from build123d import *

# Parameters (mm, degrees)
SKETCH_1_W          = 31.8
SKETCH_1_H          = 7.8
EXTRUDE_1_DEPTH     = 3.2
SKETCH_2_R          = 2.4
EXTRUDE_2_DEPTH     = 1.7
SKETCH_3_R          = 2.5
CUT_EXTRUDE_1_DEPTH = 1.8


with BuildPart() as part:
    # Эскиз1 → Бобышка-Вытянуть1 (new body)
    with BuildSketch(Plane(origin=(0, 0, 0), x_dir=(1, 0, 0), z_dir=(0, 1, 0))):
        Rectangle(SKETCH_1_W, SKETCH_1_H)
    extrude(amount=EXTRUDE_1_DEPTH)

    # Эскиз2 → Бобышка-Вытянуть2 (add)
    with BuildSketch(Plane(origin=(0, 3.2, 0), x_dir=(1, 0, 0), z_dir=(0, 1, 0))):
        with Locations(Location((-12, 0, 0), (0, 0, 270))):
            Circle(SKETCH_2_R)
        with Locations(Location((-4.126, 0, 0), (0, 0, 270))):
            Circle(SKETCH_2_R)
        with Locations(Location((3.748, 0, 0), (0, 0, 270))):
            Circle(SKETCH_2_R)
        with Locations(Location((11.622, 0, 0), (0, 0, 270))):
            Circle(SKETCH_2_R)
    extrude(amount=EXTRUDE_2_DEPTH)

    # Эскиз3 → Вырез-Вытянуть1 (cut)
    with BuildSketch(Plane.XZ):
        with Locations(Location((-12, 0, 0), (0, 0, 270))):
            Circle(SKETCH_3_R)
        with Locations(Location((-4.126, 0, 0), (0, 0, 270))):
            Circle(SKETCH_3_R)
        with Locations(Location((3.748, 0, 0), (0, 0, 270))):
            Circle(SKETCH_3_R)
        with Locations(Location((11.622, 0, 0), (0, 0, 270))):
            Circle(SKETCH_3_R)
    extrude(amount=-CUT_EXTRUDE_1_DEPTH, mode=Mode.SUBTRACT)


solid = part.part
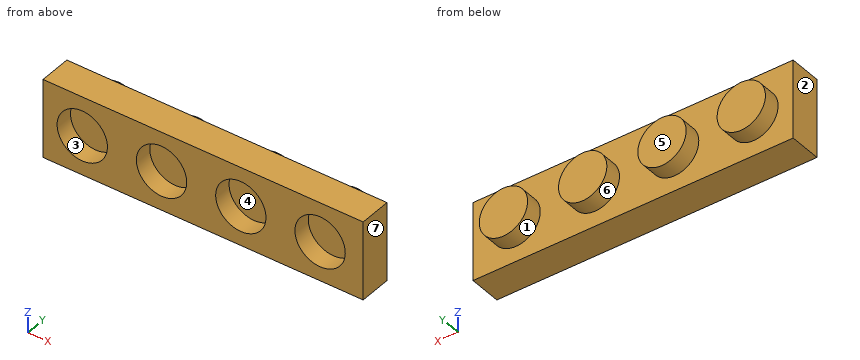
Source: CAD feature listing. Evaluate the final solid. Frame: model axes, mm. Face numbers are marked on the shaded views. A direction names the side the tool comes from. Round coordinates to 2 decimals unless told otherwise and drop trailing zeros. Loops run counter-clockwise (first coordinate to the right, second up) from the corner with the lowest first, then second, coordinate; pieces in that order, holes last. Notation, with made-up numbers: M -6.5,9.5 L 10.5,9.5 A24 ccw 10.5,23.5 Z; hole C 82,-1.75 d8. An arc over 180 degrees is marked long. Return JSON: item names as keys, results as strings. Group by question number.
1. Section query C-C on y = 4.5. Output: boundary loops of the cut face in (x, z), and give its area (3 significant figures).
2. Section query A-A on x = -12. Output: boundary loops of the cut face in (y, z).
3. Pin query (flat end, axial travel): pin 1 (1.5 mm diameter, centred on x = -4.5, z = -1, fed in from -Y). Return the tip coordinate at first contact, or that it passes through.
4. Material intervals for line 1 along X through (y, z) = (1, 0); line 2 along X through (y, z) = (3.55, 2); line 3 along X through (y, z) = (0.95, -0.75), sorted ascending. Write a range as from..to.
5. Section query D-D on x = -5.5. Output: boundary loops of the cut face in (y, z), and give its area (3 significant figures).
6. Mould query, pull axis X, two halves, no side actions, for the marked faces 4, 5, 6 and 7. Classes: released by +X, released by -X, zero draft, split by the parting line, or undercut.
7. Section query B-B on y = 0.65. Output: boundary loops of the cut face in (x, z), and give its area (4 significant figures).
8. Reachability of the marked faces 1, 2 and 3 from +Z, -Z, +X, -X, +Y, -Y: full face, straight path, thin tool, end or side. Return the list, or none.
Checks:
{
 "1": {"outline": "C -12,0 d4.8; C -4.13,0 d4.8; C 3.75,0 d4.8; C 11.62,0 d4.8", "area": "72.4 mm²"},
 "2": {"outline": "M 0,-3.9 L 3.2,-3.9 L 3.2,-2.4 L 4.9,-2.4 L 4.9,2.4 L 3.2,2.4 L 3.2,3.9 L 0,3.9 L 0,2.5 L 1.8,2.5 L 1.8,-2.5 L 0,-2.5 Z"},
 "3": {"pin 1": "stops at y = 1.8"},
 "4": {"line 1": "x = -15.9..-14.5, -9.5..-6.63, -1.63..1.25, 6.25..9.12, 14.12..15.9", "line 2": "x = -13.33..-10.67, -5.45..-2.8, 2.42..5.07, 10.3..12.95", "line 3": "x = -15.9..-14.38, -9.62..-6.51, -1.74..1.36, 6.13..9.24, 14.01..15.9"},
 "5": {"outline": "M 0,-3.9 L 3.2,-3.9 L 3.2,-1.97 L 4.9,-1.97 L 4.9,1.97 L 3.2,1.97 L 3.2,3.9 L 0,3.9 L 0,2.09 L 1.8,2.09 L 1.8,-2.09 L 0,-2.09 Z", "area": "24.1 mm²"},
 "6": {"face 4": "undercut", "face 5": "zero draft", "face 6": "undercut", "face 7": "released by +X"},
 "7": {"outline": "M -15.9,-3.9 L 15.9,-3.9 L 15.9,3.9 L -15.9,3.9 Z; hole C -12,0 d5; hole C -4.13,0 d5; hole C 3.75,0 d5; hole C 11.62,0 d5", "area": "169.5 mm²"},
 "8": {"face 1": "+Y", "face 2": "+Z, -Z, -X, +Y, -Y", "face 3": "-Y"}
}
